Source: CAD feature listing. Evaluate the final solid. Frame: model axes, mm. Face numbers are marked on the shaded views. A direction names the side the tool comes from. Round coordinates to 2 decimals unless told otherwise and drop trailing zeros. Loops run counter-clockwise (first coordinate to the right, second up) from the corner with the lowest first, then second, coordinate; pieces in that order, holes last. Notation, with made-up numbers: (-28.5, 60.5) - (-22.5, 60.5) arc R10 cw to (-22.5, 67.5) - close; hole circle Ø11 at (-17, 5.25). An arc over 180 degrees is marked (long way). One line per question, with ' | ' between items. Start each with the question number.
1. Ray query, line 1 (Y direction, x = -17, z = -23.05); line 2 (X direction, y = 3.25, z = 0.5); line 3 (Y direction, x = 12, z = 16). Return the intervals inside material, ascending.
2. Cut plane D-D (y = -9.5). Return loops of the section in (x, z).
3. Cut plane C-C (z = -12.5). Return loops of the section in (x, y), then the cut area to 3 significant figures.
4. Access query for the marked faces 1 and 2. Directions: +Z, -Z, +X, -X, +Y, -Y. A direction counts if a zero-diameter tool reaches every point of the face in a straight line with its end or side. Return the directions, or none.
5. Mould query, pull axis X, two halves, no side actions, for the marked faces 3, 4 and 5. Classes: pulls with the +X half, pulls with the -X half, needs draft (parallel to the pull), parting line crosses it, or undercut.
6. Cut plane B-B (x = -23.25). Return loops of the section in (y, z), then the cut area to 3 significant figures.
7. Cut plane A-A (z = 0). Return loops of the section in (x, y).
8. Pin query (flat end, axial travel): pin 1 (7 mm diameter, centred on x = -17, y = -4.79, fed in from +Z); pin 2 (5 mm diameter, centred on y = -4.79, z = -11.65, fed in from +X); pin 3 (1 mm diameter, centred on y = -10, z = 14, fed in from +X). Return the tip coordinate at first contact, or that it passes through.
```python
from build123d import *

# Parameters (mm, degrees)
SKETCH1_W                = 58.5
SKETCH1_H                = 43.3
SKETCH1_R                = 16.5
BOSS_EXTRUDE1_DEPTH      = 7
M5_CLEARANCE_HOLE1_D     = 5.8
M5_CLEARANCE_HOLE1_DEPTH = 7
SKETCH5_W                = 58.5
SKETCH5_H                = 19.98
BOSS_EXTRUDE2_DEPTH      = 3
SKETCH6_W                = 46.3
SKETCH6_H                = 19.98
BOSS_EXTRUDE3_DEPTH      = 3
M5_CLEARANCE_HOLE2_D     = 5.5
M5_CLEARANCE_HOLE2_DEPTH = 3
M5_CLEARANCE_HOLE3_D     = 5.5
M5_CLEARANCE_HOLE3_DEPTH = 3
FILLET1_R                = 1
FILLET2_R                = 1


with BuildPart() as part:
    # Sketch1 → Boss-Extrude1 (new body)
    with BuildSketch(Plane(origin=(0, 0, 0), x_dir=(1, 0, 0), z_dir=(0, 1, 0))):
        Rectangle(SKETCH1_W, SKETCH1_H)
        Circle(SKETCH1_R, mode=Mode.SUBTRACT)
    extrude(amount=BOSS_EXTRUDE1_DEPTH)

    # M5 Clearance Hole1
    with Locations(Plane(origin=(0, 7, 0), x_dir=(1, 0, 0), z_dir=(0, 1, 0))):
        with Locations((-23.25, 0), (23.25, 0)):
            Hole(M5_CLEARANCE_HOLE1_D / 2, depth=M5_CLEARANCE_HOLE1_DEPTH)

    # Sketch5 → Boss-Extrude2 (add)
    with BuildSketch(Plane(origin=(0, 0, -21.65), x_dir=(-1, 0, 0), z_dir=(0, 0, -1))):
        with Locations((0, -2.99)):
            Rectangle(SKETCH5_W, SKETCH5_H)
    extrude(amount=BOSS_EXTRUDE2_DEPTH)

    # Sketch6 → Boss-Extrude3 (add)
    with BuildSketch(Plane.ZY.offset(29.25)):
        with Locations((-1.5, -2.99)):
            Rectangle(SKETCH6_W, SKETCH6_H)
    extrude(amount=BOSS_EXTRUDE3_DEPTH)

    # M5 Clearance Hole2
    with Locations(Plane.XY.offset(-21.65)):
        with Locations((-17, -4.79), (17, -4.79)):
            Hole(M5_CLEARANCE_HOLE2_D / 2, depth=M5_CLEARANCE_HOLE2_DEPTH)

    # M5 Clearance Hole3
    with Locations(Plane(origin=(-29.25, 0, 0), x_dir=(0, 0, -1), z_dir=(1, 0, 0))):
        with Locations((-11.65, -4.79), (11.65, -4.79)):
            Hole(M5_CLEARANCE_HOLE3_D / 2, depth=M5_CLEARANCE_HOLE3_DEPTH)

    # Fillet1
    fillet1_edges = [part.edges().sort_by_distance(p)[0] for p in [
        (-29.25, -6.49, -21.65),
        (29.25, -6.49, -21.65),
        (0, -12.98, -21.65),
        (-29.25, -12.98, 0),
        (-29.25, -6.49, 21.65),
        (0, 0, -21.65),
        (29.25, 0, 0),
        (0, 0, 21.65),
        (-29.25, 0, 0),
    ]]
    fillet(fillet1_edges, radius=FILLET1_R)

    # Fillet2
    fillet2_edges = [part.edges().sort_by_distance(p)[0] for p in [
        (29.25, 7, -1.5),
        (-1.5, 7, -24.65),
        (29.25, -2.99, -24.65),
        (-1.5, -12.98, -24.65),
        (-32.25, -2.99, -24.65),
        (-32.25, -12.98, -1.5),
        (-32.25, -2.99, 21.65),
        (-32.25, 7, -1.5),
        (-1.5, 7, 21.65),
    ]]
    fillet(fillet2_edges, radius=FILLET2_R)


solid = part.part
```
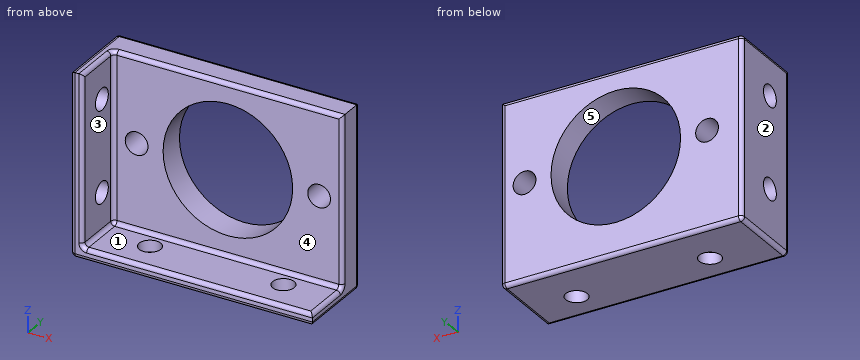
Answers follow:
1) line 1: y = -12.98 to -7.54, -2.04 to 7 | line 2: x = -32.25 to -26.11, -20.39 to -16.49, 16.49 to 20.39, 26.11 to 29.25 | line 3: y = 0 to 7
2) outline: (-32.25, -23.65) arc R1 ccw to (-31.25, -24.65) - (28.25, -24.65) arc R1 ccw to (29.25, -23.65) - (29.25, -22.65) arc R1 ccw to (28.25, -21.65) - (-28.25, -21.65) arc R1 cw to (-29.25, -20.65) - (-29.25, 20.65) arc R1 ccw to (-30.25, 21.65) - (-31.25, 21.65) arc R1 ccw to (-32.25, 20.65) - close
3) outline: (-32.25, -11.98) arc R1 ccw to (-31.25, -12.98) - (-30.25, -12.98) arc R1 ccw to (-29.25, -11.98) - (-29.25, -7.41) - (-32.25, -7.41) - close; (-32.25, -2.17) - (-29.25, -2.17) - (-29.25, -1) arc R1 cw to (-28.25, 0) - (-10.77, 0) - (-10.77, 7) - (-31.25, 7) arc R1 ccw to (-32.25, 6) - close; (10.77, 0) - (28.25, 0) arc R1 ccw to (29.25, 1) - (29.25, 6) arc R1 ccw to (28.25, 7) - (10.77, 7) - close | area: 302 mm2
4) face 1: +Z, +X, -Y | face 2: +Z, -Z, -X, +Y, -Y
5) face 3: pulls with the +X half | face 4: needs draft | face 5: undercut
6) outline: (-12.98, -23.65) arc R1 ccw to (-11.98, -24.65) - (6, -24.65) arc R1 ccw to (7, -23.65) - (7, -2.9) - (0, -2.9) - (0, -20.65) arc R1 cw to (-1, -21.65) - (-11.98, -21.65) arc R1 ccw to (-12.98, -22.65) - close; (0, 2.9) - (7, 2.9) - (7, 20.65) arc R1 ccw to (6, 21.65) - (1, 21.65) arc R1 ccw to (0, 20.65) - close | area: 322 mm2
7) outline: (-32.25, -11.98) arc R1 ccw to (-31.25, -12.98) - (-30.25, -12.98) arc R1 ccw to (-29.25, -11.98) - (-29.25, -1) arc R1 cw to (-28.25, 0) - (-26.15, 0) - (-26.15, 7) - (-31.25, 7) arc R1 ccw to (-32.25, 6) - close; (-20.35, 0) - (-16.5, 0) - (-16.5, 7) - (-20.35, 7) - close; (16.5, 0) - (20.35, 0) - (20.35, 7) - (16.5, 7) - close; (26.15, 0) - (28.25, 0) arc R1 ccw to (29.25, 1) - (29.25, 6) arc R1 ccw to (28.25, 7) - (26.15, 7) - close
8) pin 1: stops at z = -21.65 | pin 2: passes through | pin 3: stops at x = -29.25
